```python
from build123d import *

# Parameters (mm, degrees)
EXTRUDE_1_DEPTH     = 490
SKETCH_2_W          = 20
SKETCH_2_H          = 165
EXTRUDE_2_DEPTH     = 10
SKETCH_3_W          = 20
SKETCH_3_H          = 165
EXTRUDE_3_DEPTH     = 10
SKETCH_4_W          = 10
SKETCH_4_H          = 10
CUT_EXTRUDE_1_DEPTH = 527.901319034


with BuildPart() as part:
    # Эскиз1 → Бобышка-Вытянуть1 (new body)
    with BuildSketch(Plane.XY):
        Polygon((0, 0), (0, 155), (10, 155), (10, 165), (20, 165), (20, 10), (10, 10), (10, 0), align=None)
    extrude(amount=EXTRUDE_1_DEPTH)

    # Эскиз2 → Бобышка-Вытянуть2 (add)
    with BuildSketch(Plane.XY.offset(490)):
        with Locations((10, 82.5)):
            Rectangle(SKETCH_2_W, SKETCH_2_H)
    extrude(amount=EXTRUDE_2_DEPTH)

    # Эскиз3 → Бобышка-Вытянуть3 (add)
    with BuildSketch(Plane(origin=(0, 0, 0), x_dir=(-1, 0, 0), z_dir=(0, 0, -1))):
        with Locations((-10, 82.5)):
            Rectangle(SKETCH_3_W, SKETCH_3_H)
    extrude(amount=EXTRUDE_3_DEPTH)

    # Эскиз4 → Вырез-Вытянуть1 (cut, through all)
    with BuildSketch(Plane(origin=(20, 0, 0), x_dir=(0, 0, -1), z_dir=(1, 0, 0))):
        with Locations((-495, 160)):
            Rectangle(SKETCH_4_W, SKETCH_4_H)
        with Locations((5, 160)):
            Rectangle(SKETCH_4_W, SKETCH_4_H)
    extrude(amount=-CUT_EXTRUDE_1_DEPTH, mode=Mode.SUBTRACT)


solid = part.part
```
Design review of the part built by this model. Coordinates are the model's own, in mm. A direction names the side the tool comes from. Round coordinates to 2 decimals unless told otherwise and drop trailing zeros. Order: outer loops, then holes, each group sorted by start corner. A loop starts at its lowest first (then second) coordinate and runs counter-clockwise, first axis right, second up. Notation, with made-up numbers: (67, 2.25) - (122, 2.25) arc R24 ccw to (122, 32.25) - close; hole circle Ø3 at (47, 34). An arc over 180 degrees is marked (long way). Return JSON: item names as keys, results as strings.
Q1. Machinability: for faces 4 (the flat face through (10, 79, 500)), 5 (the flat face through (10, 5, 242)), 6 (the flat face through (15, 160, 490)), which of the approach directions +Z, -Z, +X, -X, +Y, -Y give a long, thin tool a straight path to every point of the face, cutting with its end or side? Answer none if there is none.
Computed values:
{"face 4": "+Z, +X, -X, +Y, -Y", "face 5": "+X, -Y", "face 6": "+Z, +X, -X, +Y"}
Q2. For pin 1 Ø11 at (x, z) = (17, 160) entering from -Y; pin 2 Ø8 at (x, y) = (17, 161.5) entering from +Z; pin 3 Ø1 at (x, z) = (8.5, 176.5) entering from +Y, all flat-tipped, find the tip position at first contact; note any pin that passes through.
Computed values:
{"pin 1": "stops at y = 10", "pin 2": "stops at z = 490", "pin 3": "stops at y = 155"}
Q3. Consider section A-A on z = 285. Write out the cut boundary in (x, y), plus the area to 3 significant figures.
Computed values:
{"outline": "(0, 0) - (10, 0) - (10, 10) - (20, 10) - (20, 165) - (10, 165) - (10, 155) - (0, 155) - close", "area": "3,100 mm2"}
Q4. Consider section B-B on x = 5.75. Write out the cut boundary in (y, z), plus the area to 4 significant figures.
Computed values:
{"outline": "(0, -10) - (155, -10) - (155, 500) - (0, 500) - close", "area": "79,050 mm2"}
Q5. The part is to be moulded in two halves that separate along Z. For faces 1 (the flat face through (15, 10, 242)), 2 (the flat face through (10, 160, 242)), 3 (the flat face through (15, 160, 0)), say which applies: pulls with the +Z half, pulls with the -Z half, needs draft (parallel to the pull), parting line crosses it, or undercut.
Computed values:
{"face 1": "undercut", "face 2": "needs draft", "face 3": "pulls with the -Z half"}
Q6. Wall thickness on L1, parallel to Z at x = 13.5, y = 7.5; L2, parallel to Y at x = 8, z = 192; L3, parallel to Y at x = 18.25, z = 339: over which ranges is each line inside the solid? List them lowest first. Write a range as [from, to].
Computed values:
{"L1": "z = [-10, 0], [490, 500]", "L2": "y = [0, 155]", "L3": "y = [10, 165]"}
